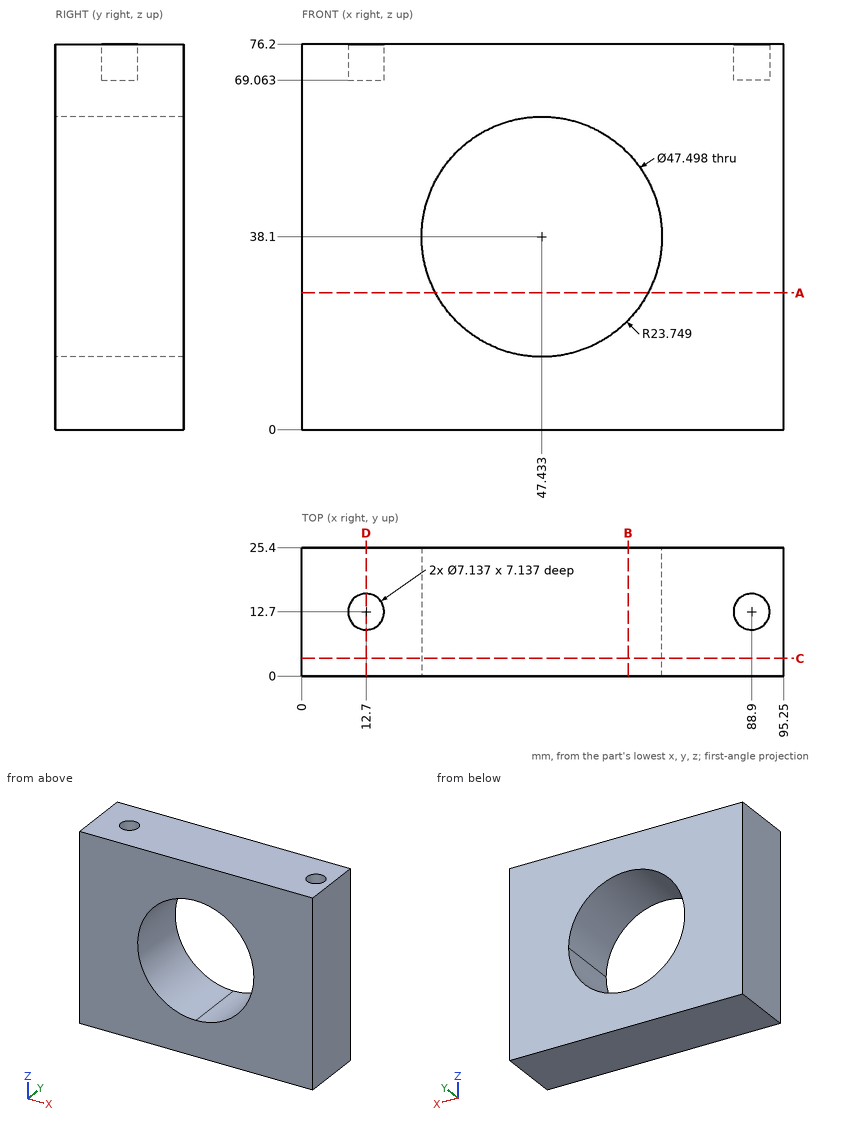
Could you check a few things on this drawing? It's one solid part, dimensions in mm from its lowest x, y, z. Coordinates: 2 decimals unless noted, no trailing zeros. Write each loop counter-clockwise with the first axis right and the second up, starting at its lowest first coordinate (ties: lowest second). Pieces come first, ordered by that corner, then holes.
Q1. Please list where these lines run through material, in increasing order: L1, parallel to Y at x = 12.7, z = 72.5; L2, parallel to X at y = 20.75, z = 45.5; L3, parallel to X at y = 6.5, z = 36.
Results found:
L1: y = 0 to 9.13, 16.27 to 25.4
L2: x = 0 to 24.87, 70 to 95.25
L3: x = 0 to 23.78, 71.09 to 95.25
Q2. Imagine slicing it at A-A, the plane z = 27. List the corners of the cut face in (x, y) for me, plus the area to 3 significant figures.
Results found:
outline: (0, 0) - (26.44, 0) - (26.44, 25.4) - (0, 25.4) - close; (68.43, 0) - (95.25, 0) - (95.25, 25.4) - (68.43, 25.4) - close
area: 1,350 mm2
Q3. Imagine slicing it at B-B, the plane x = 64.5. List the corners of the cut face in (y, z) for me (1 decimal), plus the area to 3 significant figures.
Results found:
outline: (0, 0) - (25.4, 0) - (25.4, 21.6) - (0, 21.6) - close; (0, 54.6) - (25.4, 54.6) - (25.4, 76.2) - (0, 76.2) - close
area: 1,100 mm2
Q4. For P1, Ø4, axis at y = 3, z = 65.5, coming from the -X side; P2, Ø2, axis at x = 14, y = 13, coming from the +Z side, each with a flat end and sliding along its axis, tell me the tip position at first contact or that it passes through.
Results found:
P1: stops at x = 0
P2: stops at z = 69.06
Q5. Imagine slicing it at C-C, the plane y = 3.5. List the corners of the cut face in (x, z) for me.
Results found:
outline: (0, 0) - (95.25, 0) - (95.25, 76.2) - (0, 76.2) - close; hole (47.47, 14.35) arc R23.75 ccw to (71.18, 38.1) arc R23.75 ccw (long way) to start
Q6. Imagine slicing it at D-D, the plane x = 12.7. List the corners of the cut face in (y, z) for me.
Results found:
outline: (0, 0) - (25.4, 0) - (25.4, 76.2) - (16.27, 76.2) - (16.27, 69.06) - (9.13, 69.06) - (9.13, 76.2) - (0, 76.2) - close
